Can you work these out from the model? Positions are in its coordinate system, mm. A direction names the side the tool comes from. Give positions to 0.01 mm unless a question says otherwise; leave off trailing zeros. Loops run counter-clockwise (first coordinate to the right, second up) from the corner with the lowest first, then second, coordinate; pieces in that order, holes last. Notation, with made-up numbers: (31.25, -33.5) - (84.25, -33.5) arc R18 cw to (84.25, -2.5) - close; hole circle Ø4 at (53, 16). An arc over 180 degrees is marked (long way). Answer as a JSON object with one key per item and string values.
```python
from build123d import *

# Parameters (mm, degrees)
BOSS_EXTRUDE1_DEPTH = 25.4
SKETCH2_R           = 2.54
CUT_EXTRUDE1_DEPTH  = 91.02678768
SKETCH3_W           = 4.7625
SKETCH3_H           = 50.8
CUT_EXTRUDE2_DEPTH  = 91.02678768
SKETCH4_W           = 44.45
SKETCH4_H           = 19.05
CUT_EXTRUDE3_DEPTH  = 91.02678768
FILLET1_R           = 5.08
SKETCH6_R           = 4.064
CUT_EXTRUDE5_DEPTH  = 7.62


with BuildPart() as part:
    # Sketch1 → Boss-Extrude1 (new body)
    with BuildSketch(Plane.XY):
        Polygon((0, 0), (0, 50.8), (25.4, 50.8), (25.4, 25.4), (69.85, 25.4), (69.85, 0), align=None)
    extrude(amount=BOSS_EXTRUDE1_DEPTH)

    # Sketch2 → Cut-Extrude1 (cut, through all)
    with BuildSketch(Plane.XY.offset(25.4)):
        with Locations((12.7, 38.1)):
            Circle(SKETCH2_R)
        with Locations((12.7, 12.7)):
            Circle(SKETCH2_R)
        with Locations((38.1, 12.7)):
            Circle(SKETCH2_R)
        with Locations((63.5, 12.7)):
            Circle(SKETCH2_R)
    extrude(amount=-CUT_EXTRUDE1_DEPTH, mode=Mode.SUBTRACT)

    # Sketch3 → Cut-Extrude2 (cut, through all)
    with BuildSketch(Plane.XY.offset(25.4)):
        with Locations((2.38125, 25.4)):
            Rectangle(SKETCH3_W, SKETCH3_H)
    extrude(amount=-CUT_EXTRUDE2_DEPTH, mode=Mode.SUBTRACT)

    # Sketch4 → Cut-Extrude3 (cut, through all)
    with BuildSketch(Plane.XZ):
        with Locations((47.625, 15.875)):
            Rectangle(SKETCH4_W, SKETCH4_H)
    extrude(amount=-CUT_EXTRUDE3_DEPTH, mode=Mode.SUBTRACT)

    # Fillet1
    fillet1_edges = [part.edges().sort_by_distance(p)[0] for p in [
        (25.4, 25.4, 3.175),
        (25.4, 12.7, 6.35),
    ]]
    fillet(fillet1_edges, radius=FILLET1_R)

    # Sketch6 → Cut-Extrude5 (cut)
    with BuildSketch(Plane(origin=(0, 0, 0), x_dir=(-1, 0, 0), z_dir=(0, 0, -1))):
        with Locations((-12.7, 38.1)):
            Circle(SKETCH6_R)
    extrude(amount=-CUT_EXTRUDE5_DEPTH, mode=Mode.SUBTRACT)


solid = part.part
```
1) I need wall thicknesses on L1, parallel to Y at x = 12.7, z = 19; L2, parallel to Y at x = 63.5, z = 2.25; L3, parallel to Y at x = 12.7, z = 6. Which ranges of each line are inside material? Lowest first, please.
Check sheet entries:
{"L1": "0 to 10.16, 15.24 to 35.56, 40.64 to 50.8", "L2": "0 to 10.16, 15.24 to 25.4", "L3": "0 to 10.16, 15.24 to 34.04, 42.16 to 50.8"}
2) Which directions (+Z, -Z, +X, -X, +Y, -Y) give clear straight access to the entire face, cutting with the end or side of a thin tool? Please do faces 1 (the flat face through (25.4, 31, 15)), 2 (the flat face through (50, 25.4, 3)), 3 (the flat face through (50, 13, 6.35)), 4 (the cylindrical face through (16.76, 38.28, 3.76)), 5 (the cylindrical face through (65.923, 13.463, 3.219)).
Check sheet entries:
{"face 1": "+Z, +X, +Y", "face 2": "+Z, -Z, +X, +Y", "face 3": "+Z, +X, +Y, -Y", "face 4": "-Z", "face 5": "+Z, -Z"}
3) If we mould it in two halves opening along X, with no side actions, what happens to faces 6 (the flat face through (4.762, 25, 13)), 7 (the flat face through (15, 36, 7.62)), 8 (the flat face through (15, 26, 25.4))? For each: released by +X, released by -X, zero draft, split by the parting line, or undercut.
Check sheet entries:
{"face 6": "released by -X", "face 7": "undercut", "face 8": "zero draft"}
4) Imagine slicing it at C-C on z = 15.25. Write out the boundary of the cut face in (x, y).
Check sheet entries:
{"outline": "(4.76, 0) - (25.4, 0) - (25.4, 50.8) - (4.76, 50.8) - close; hole circle Ø5.08 at (12.7, 12.7); hole circle Ø5.08 at (12.7, 38.1)"}
5) I'm going to push flat-ended pins straight in: P1, Ø2, axis at x = 31.5, z = 9, coming from the -Y side; P2, Ø7, axis at x = 44, z = 4.5, coming from the +Y side; P3, Ø7.5, axis at x = 46.5, y = 18, coming from the +Z side; P4, Ø6.5, axis at x = 12.7, y = 38.1, coming from the -Z side. Where does each tip first touch, or does it pass through?
Check sheet entries:
{"P1": "through", "P2": "y = 25.4", "P3": "z = 6.35", "P4": "z = 7.62"}
6) Imagine slicing it at A-A on x = 63.5. Write out the boundary of the cut face in (y, z), and give its area (3 significant figures).
Check sheet entries:
{"outline": "(0, 0) - (10.16, 0) - (10.16, 6.35) - (0, 6.35) - close; (15.24, 0) - (25.4, 0) - (25.4, 6.35) - (15.24, 6.35) - close", "area": "129 mm2"}
7) Imagine slicing it at B-B on y = 38.1. Write out the boundary of the cut face in (x, z), and give its area (3 significant figures).
Check sheet entries:
{"outline": "(4.76, 0) - (8.64, 0) - (8.64, 7.62) - (10.16, 7.62) - (10.16, 25.4) - (4.76, 25.4) - close; (15.24, 7.62) - (16.76, 7.62) - (16.76, 0) - (25.4, 0) - (25.4, 25.4) - (15.24, 25.4) - close", "area": "372 mm2"}
8) Imagine slicing it at D-D on x = 12.7. Write out the boundary of the cut face in (y, z).
Check sheet entries:
{"outline": "(0, 0) - (10.16, 0) - (10.16, 25.4) - (0, 25.4) - close; (15.24, 0) - (34.04, 0) - (34.04, 7.62) - (35.56, 7.62) - (35.56, 25.4) - (15.24, 25.4) - close; (40.64, 7.62) - (42.16, 7.62) - (42.16, 0) - (50.8, 0) - (50.8, 25.4) - (40.64, 25.4) - close"}
